Design review of the part built by this model. Coordinates are the model's own, in mm. A direction names the side the tool comes from. Coordinates: 2 decimals unless noted, no trailing zeros. Order: outer loops, then holes, each group sorted by start corner. A loop starts at its lowest first (then second) coordinate and runs counter-clockwise, first axis right, second up. Notation, with made-up numbers: (-19.5, -32) -> (18.5, -32) arc R25 cw to (18.5, -14) -> close; hole circle Ø3 at (-24.75, 83.5). An arc over 180 degrees is marked (long way). Use a Markdown table: item, result. Add a question column.
Q1. Add section A-A (z = -8.5). State the section outline as (x, y) points (3 decimals), then the cut area to 3 significant figures.
Q2. Add section B-B (y = 17). State the section outline as (x, z) points (3 decimals), then the cut area to 3 significant figures.
Q3. Wall thickness on probe 1 along X at (y, z) = (16.5, -1.5) (3 decimals); probe 2 along X at (y, z) = (1.5, 2.25); probe 3 along Z at (x, y) = (-2, 40.5) (3 decimals): over which ranges is each line inside the solid? List them lowest first.
Q4. Machinability: for faces 4 (the face through (0.119, -45.453, 0.088)), 5 (the face through (2.705, 0, 2)), 6 (the face through (22.225, 2, -5)), which of the approach directions +Z, -Z, +X, -X, +Y, -Y give a long, thin tool a straight path to every point of the face, cutting with its end or side? Answer none if there is none.
Q5. Add section D-D (x = 9). State the section outline as (y, z) points (3 decimals), then the cut area to 3 significant figures.
Q6. Insertion check: pin 1 (13.5 mm diameter, centred on x = -8, y = -6, fed in from -Z); pin 2 (3 mm diameter, centred on x = -20, z = -4, fed in from +Y). Each pin has a flat end and moves straight along its axis. Give the tip position at first contact, or say it passes through.
Q7. The part is to be moulded in two halves that separate along X. For faces 1 (the face through (-22.225, 2, -5)), 2 (the face through (-1.763, 47.772, 0.147)), 3 (the face through (25.4, -1, -3)), say which applies: pulls with the +X half, pulls with the -X half, needs draft (parallel to the pull), parting line crosses it, or undercut.
from build123d import *

# Parameters (mm, degrees)
F0_W     = 50.8
F0_H     = 101.6
F1_DEPTH = 3.175
F2_W     = 3.175
F2_H     = 101.6
F3_DEPTH = 9.525
F5_DEPTH = 50.8
F7_DEPTH = 25.4


with BuildPart() as f1:
    # F0 (on Top) → F1 (new body)
    with BuildSketch(Plane.XY):
        Rectangle(F0_W, F0_H)
    extrude(amount=F1_DEPTH)

    # F2 (on face) → F3 (join)
    with BuildSketch(Plane(origin=(0, 0, 0), x_dir=(1, 0, 0), z_dir=(0, 0, -1))):
        with Locations((-23.8125, 0)):
            Rectangle(F2_W, F2_H)
        with Locations((23.8125, 0)):
            Rectangle(F2_W, F2_H)
    extrude(amount=F3_DEPTH)

    # F4 (on face) → F5 (cut)
    with BuildSketch(Plane.YZ.offset(25.4)):
        Polygon((-28.8029547439, -9.525), (-50.8, 3.175), (-50.8, -9.525), align=None)
        Polygon((50.8, -9.525), (50.8, 3.175), (38.1, -9.525), align=None)
    extrude(amount=-F5_DEPTH, mode=Mode.SUBTRACT)

    # F6 (on face) → F7 (cut)
    with BuildSketch(Plane.XY.offset(3.175)):
        with BuildLine():
            Line((-0.4691980296, 0), (-0.4691980296, 6.35))
            ThreePointArc((-0.4691980296, 6.35), (-2.639728339, 5.492201583), (-3.6374224509, 3.3823138118))
            Line((-3.6374224509, 3.3823138118), (-3.6377601108, 2.9729125496))
            ThreePointArc((-3.6377601108, 2.9729125496), (-2.6416387475, 0.8595893825), (-0.4691980296, 0))
        make_face()
        with BuildLine():
            ThreePointArc((2.7045093513, 3.2655895149), (1.7436059936, 5.4518670042), (-0.4691980296, 6.35))
            Line((-0.4691980296, 6.35), (-0.4691980296, 0))
            ThreePointArc((-0.4691980296, 0), (1.7436059936, 0.8981329958), (2.7045093513, 3.0844104851))
            Line((2.7045093513, 3.0844104851), (2.7045093513, 3.2655895149))
        make_face()
        with BuildLine():
            Line((-0.4691980296, 0), (-0.4691980296, -6.35))
            ThreePointArc((-0.4691980296, -6.35), (1.7436059936, -5.4518670042), (2.7045093513, -3.2655895149))
            Line((2.7045093513, -3.2655895149), (2.7045093513, -3.0844104851))
            ThreePointArc((2.7045093513, -3.0844104851), (1.7436059936, -0.8981329958), (-0.4691980296, 0))
        make_face()
        with BuildLine():
            ThreePointArc((-3.6429054106, -3.2655895149), (-2.6820020528, -5.4518670042), (-0.4691980296, -6.35))
            Line((-0.4691980296, -6.35), (-0.4691980296, 0))
            ThreePointArc((-0.4691980296, 0), (-2.6801234201, -0.8963087269), (-3.6427516628, -3.0791754847))
            Line((-3.6427516628, -3.0791754847), (-3.6429054106, -3.2655895149))
        make_face()
        with BuildLine():
            ThreePointArc((-3.6427516628, -3.0791754847), (-3.6441969498, -3.1723813712), (-3.6429054106, -3.2655895149))
            Line((-3.6429054106, -3.2655895149), (-3.6427516628, -3.0791754847))
        make_face()
        with BuildLine():
            ThreePointArc((2.7045093513, 3.0844104851), (1.7436059936, 0.8981329958), (-0.4691980296, 0))
            ThreePointArc((-0.4691980296, 0), (1.7436059936, -0.8981329958), (2.7045093513, -3.0844104851))
            Line((2.7045093513, -3.0844104851), (2.7045093513, 3.0844104851))
        make_face()
        with BuildLine():
            ThreePointArc((-3.6427516628, -3.0791754847), (-2.6801234201, -0.8963087269), (-0.4691980296, 0))
            ThreePointArc((-0.4691980296, 0), (-2.6416387475, 0.8595893825), (-3.6377601108, 2.9729125496))
            Line((-3.6377601108, 2.9729125496), (-3.6427516628, -3.0791754847))
        make_face()
    extrude(amount=-F7_DEPTH, mode=Mode.SUBTRACT)


solid = f1.part
Established:
| question | item | result |
|---|---|---|
| 1 | outline | (-25.4, -30.578) -> (-22.225, -30.578) -> (-22.225, 39.125) -> (-25.4, 39.125) -> close; (22.225, -30.578) -> (25.4, -30.578) -> (25.4, 39.125) -> (22.225, 39.125) -> close |
| 1 | area | 443 mm^2 |
| 2 | outline | (-25.4, -9.525) -> (-22.225, -9.525) -> (-22.225, 0) -> (22.225, 0) -> (22.225, -9.525) -> (25.4, -9.525) -> (25.4, 3.175) -> (-25.4, 3.175) -> close |
| 2 | area | 222 mm^2 |
| 3 | probe 1 | -25.4 to -22.225, 22.225 to 25.4 |
| 3 | probe 2 | -25.4 to -3.64, 2.7 to 25.4 |
| 3 | probe 3 | 0 to 3.175 |
| 4 | face 4 | -Z, +X, -X, -Y |
| 4 | face 5 | +Z, -Z |
| 4 | face 6 | -Z, +Y, -Y |
| 5 | outline | (-50.8, 3.175) -> (-45.301, 0) -> (47.625, 0) -> (50.8, 3.175) -> close |
| 5 | area | 309 mm^2 |
| 6 | pin 1 | z = 0 |
| 6 | pin 2 | through |
| 7 | face 1 | undercut |
| 7 | face 2 | needs draft |
| 7 | face 3 | pulls with the +X half |
